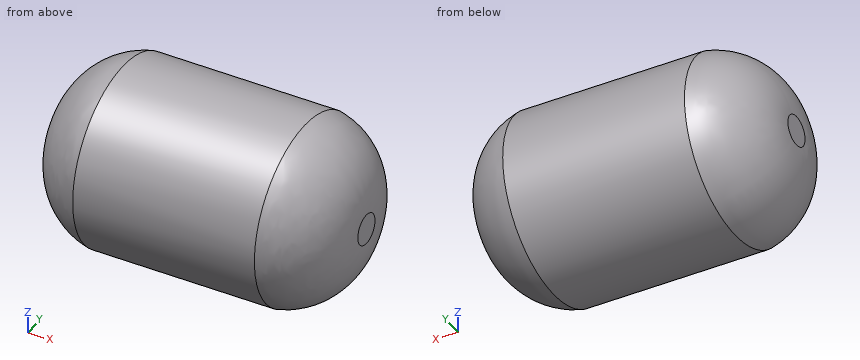
```python
from build123d import *


# Read off the part's stored shape, not the designer's step: Revolve-Thin1
with BuildPart() as part:
    # Revolve-Thin1 outline → Revolve-Thin1 (revolve)
    with BuildSketch(Plane.YX):
        with BuildLine():
            Line((60, 0), (60, 60))
            ThreePointArc((60, 60), (42.192905916, 88.991132396), (10, 100))
            Line((10, 100), (0, 100))
            Line((0, 100), (0, 99))
            Line((0, 99), (10.007910772, 99))
            ThreePointArc((10.007910772, 99), (41.525060748, 88.244744032), (59, 59.896326585))
            Line((59, 59.896326585), (59, 0))
            Line((59, 0), (60, 0))
        make_face()
    revolve_thin1 = revolve(axis=Axis((0, 0, 0), (1, 0, 0)))

    # Mirror1: Revolve-Thin1 across plane
    add(revolve_thin1.mirror(Plane(origin=(0, 0, -59), x_dir=(0, 0, 1), z_dir=(-1, 0, 0))))


solid = part.part
```
Could you check a few things on this model? Use its own coordinates, in mm. Round coordinates to 2 decimals unless told otherwise and drop trailing zeros. Loops run counter-clockwise (first coordinate to the right, second up) from the corner with the lowest first, then second, coordinate; pieces in that order, holes last.
Q1. Please list where these lines run through material, in increasing order: L1, parallel to Z at x = -41.5, y = 0; L2, parallel to X at y = 3.5, z = 12; L3, parallel to X at y = 1, z = -44.
Q2. I want a section at A-A (x = -56). Write out the boundary of the cut face in (y, z).
Q3. For P1, Ø10, axis at y = -31.5, z = 26.5, coming from the -X side; P2, Ø3, axis at x = -66, y = 17, coming from the -Z side; P3, Ø6, axis at y = -3.5, z = -0.5, coming from the +X side; P4, Ø10, axis at x = -55.5, z = -0.5, coming from the -Y side, each with a flat end and sliding along its axis, tell me the tip position at first contact or that it passes through.
Answer below:
1. L1: z = -60 to -59, 59 to 60
1. L2: x = -99.98 to -98.98, 98.98 to 99.98
1. L3: x = -87.46 to -86.12, 86.12 to 87.46
2. outline: circle Ø120 at (0, 0); hole circle Ø118 at (0, 0)
3. P1: stops at x = -93.13
3. P2: stops at z = -56.5
3. P3: stops at x = 100
3. P4: stops at y = -60
